Autodesk Inventor part; units mm, degrees
ref_plane "YZ Plane" through (0, 0, 0) normal (1, 0, 0) x (0, 1, 0)
ref_plane "XZ Plane" through (0, 0, 0) normal (0, 1, 0) x (-1, 0, 0)
ref_plane "XY Plane" through (0, 0, 0) normal (0, 0, 1) x (1, 0, 0)
sketch "スケッチ1" plane through (0, 0, 0) normal (1, 0, 0) x (0, 1, 0)
  point P0 (0, 0)
sketch "スケッチ2" plane through (0, 0, 0) normal (0, 0, 1) x (1, 0, 0)
  line L0 (-11.1, 11.1) -> (11.1, 11.1)
  line L1 (11.1, 11.1) -> (11.1, -11.1)
  line L2 (11.1, -11.1) -> (-11.1, -11.1)
  line L3 (-11.1, -11.1) -> (-11.1, 11.1)
  line L4 (-11.1, 11.1) -> (11.1, -11.1) construction
  line L5 (11.1, 11.1) -> (-11.1, -11.1) construction
  line L6 (-13.5, -13.5) -> (13.5, -13.5)
  line L7 (13.5, -13.5) -> (13.5, 13.5)
  line L8 (13.5, 13.5) -> (-13.5, 13.5)
  line L9 (-13.5, 13.5) -> (-13.5, -13.5)
  line L10 (-13.5, -13.5) -> (13.5, 13.5) construction
  line L11 (13.5, -13.5) -> (-13.5, 13.5) construction
  point P0 (0, 0)
  dimension "d0" = 22.2
  dimension "d1" = 22.2
  dimension "d2" = 27
  dimension "d3" = 27
extrude "押し出し1" add sketch "スケッチ2" along normal blind 15
sketch "スケッチ3" plane through (-13.5, 13.5, 0) normal (0, 1, 0) x (1, 0, 0)
  circle A0 centre (13.5, -10) radius 1.7
  point P0 (13.5, 0)
  dimension "d6" = 3.4
extrude "押し出し2" cut sketch "スケッチ3" against normal blind 30
sketch "スケッチ4" plane through (0, 0, 0) normal (0, 0, -1) x (-1, 0, 0)
  line L0 (22, 22) -> (-22, 22)
  line L1 (-22, 22) -> (-22, -22)
  line L2 (-22, -22) -> (22, -22)
  line L3 (22, -22) -> (22, 22)
  line L4 (22, 22) -> (-22, -22) construction
  line L5 (-22, 22) -> (22, -22) construction
  point P0 (0, 0)
  dimension "d9" = 44
  dimension "d10" = 44
extrude "押し出し3" add sketch "スケッチ4" along normal blind 3
sketch "スケッチ5" plane through (0, 0, 0) normal (0, 0, 1) x (1, 0, 0)
  circle A0 centre (0, 17.75) radius 2.25
  circle A1 centre (0, -17.75) radius 2.25
  point P0 (0, 0)
  dimension "d13" = 4.5
  dimension "d14" = 4.5
extrude "押し出し4" cut sketch "スケッチ5" against normal blind 3
sketch "スケッチ6" plane through (0, 0, 0) normal (0, 0, 1) x (1, 0, 0)
  line L0 (-22, 22) -> (22, 22)
  line L1 (22, 22) -> (11, 22)
  line L2 (22, 22) -> (22, 11)
  line L3 (22, 11) -> (11, 22)
  line L4 (22, -22) -> (-22, -22)
  line L5 (22, -22) -> (22, -11)
  line L6 (22, 22) -> (22, -22)
  line L7 (22, -22) -> (11, -22)
  line L8 (11, -22) -> (22, -11)
  line L9 (-22, -22) -> (-22, 22)
  line L10 (-22, 22) -> (-11, 22)
  line L11 (-22, 22) -> (-22, 11)
  line L12 (-22, 11) -> (-11, 22)
  line L13 (-22, -22) -> (-22, -11)
  line L14 (-22, -22) -> (-11, -22)
  line L15 (-22, -11) -> (-11, -22)
  point P0 (0, 0)
  dimension "d17" = 11
  dimension "d18" = 11
  dimension "d19" = 11
  dimension "d20" = 11
  dimension "d21" = 11
  dimension "d22" = 11
  dimension "d23" = 11
extrude "押し出し5" cut sketch "スケッチ6" against normal blind 3 contours L0 L12 L9 | L0 L2 L3 | L15 L4 L9 | L5 L4 L8
fillet "フィレット1" radius 3 4 edges at (13.5, -13.5, 7.5) (13.5, 13.5, 7.5) (-13.5, -13.5, 7.5) (-13.5, 13.5, 7.5)
fillet "フィレット2" radius 1 4 edges at (-11.1, 11.1, 7.5) (-11.1, -11.1, 7.5) (11.1, 11.1, 7.5) (11.1, -11.1, 7.5)
properties part number "rod_fixture_vp16"
Design review of the part built by this model. Coordinates are the model's own, in mm. A direction names the side the tool comes from. Round coordinates to 2 decimals unless told otherwise and drop trailing zeros. Write each loop counter-clockwise with the first axis right and the second up, starting at its lowest first coordinate (ties: lowest second). Pieces come first, ordered by that corner, then holes. Notation, with made-up numbers: (81, 33.5) -> (116, 33.5) arc R22 ccw to (116, 68.5) -> close; hole circle Ø1 at (82, -8). An arc over 180 degrees is marked (long way). One line per question, with ' | ' between items.
(1) Take a section at A-A, the plane x = 0. State the section outline as (y, z) points, and give its area (3 significant figures).
Result sheet:
outline: (-22, -3) -> (-20, -3) -> (-20, 0) -> (-22, 0) -> close; (-15.5, -3) -> (15.5, -3) -> (15.5, 0) -> (13.5, 0) -> (13.5, 8.3) -> (11.1, 8.3) -> (11.1, 0) -> (-11.1, 0) -> (-11.1, 8.3) -> (-13.5, 8.3) -> (-13.5, 0) -> (-15.5, 0) -> close; (-13.5, 11.7) -> (-11.1, 11.7) -> (-11.1, 15) -> (-13.5, 15) -> close; (11.1, 11.7) -> (13.5, 11.7) -> (13.5, 15) -> (11.1, 15) -> close; (20, -3) -> (22, -3) -> (22, 0) -> (20, 0) -> close | area: 161 mm2
(2) Insertion check: P1, Ø4, axis at y = -8.5, z = 11.5, coming from the +X side; P2, Ø5, axis at x = 9, z = 4, coming from the +Y side; P3, Ø4.5, axis at y = -3, z = 8, coming from the -X side. Each pin has a flat end and moves straight along its axis. Give the tip position at first contact, or say it passes through.
Result sheet:
P1: x = 13.5 | P2: y = 13.5 | P3: x = -13.5
(3) Take a section at D-D, the plane z = 10. State the section outline as (x, y) points, and give its area (3 significant figures).
Result sheet:
outline: (-13.5, -10.5) arc R3 ccw to (-10.5, -13.5) -> (-1.7, -13.5) -> (-1.7, -11.1) -> (-10.1, -11.1) arc R1 cw to (-11.1, -10.1) -> (-11.1, 10.1) arc R1 cw to (-10.1, 11.1) -> (-1.7, 11.1) -> (-1.7, 13.5) -> (-10.5, 13.5) arc R3 ccw to (-13.5, 10.5) -> close; (1.7, -13.5) -> (10.5, -13.5) arc R3 ccw to (13.5, -10.5) -> (13.5, 10.5) arc R3 ccw to (10.5, 13.5) -> (1.7, 13.5) -> (1.7, 11.1) -> (10.1, 11.1) arc R1 cw to (11.1, 10.1) -> (11.1, -10.1) arc R1 cw to (10.1, -11.1) -> (1.7, -11.1) -> close | area: 213 mm2
(4) Wall thickness on line 1 (Y direction, x = 0, z = -1.5); line 2 (X direction, y = 2, z = 6.75); line 3 (Z direction, x = 0, y = -11.65): over which ranges is each line inside the solid? List them lowest first. Write a range as [from, to].
Result sheet:
line 1: [-22, -20], [-15.5, 15.5], [20, 22] | line 2: [-13.5, -11.1], [11.1, 13.5] | line 3: [-3, 8.3], [11.7, 15]
(5) Take a section at C-C, the plane z = 1.5. State the section outline as (x, y) points, and give its area (3 significant figures).
Result sheet:
outline: (-13.5, -10.5) arc R3 ccw to (-10.5, -13.5) -> (10.5, -13.5) arc R3 ccw to (13.5, -10.5) -> (13.5, 10.5) arc R3 ccw to (10.5, 13.5) -> (-10.5, 13.5) arc R3 ccw to (-13.5, 10.5) -> close; hole (-11.1, -10.1) arc R1 ccw to (-10.1, -11.1) -> (10.1, -11.1) arc R1 ccw to (11.1, -10.1) -> (11.1, 10.1) arc R1 ccw to (10.1, 11.1) -> (-10.1, 11.1) arc R1 ccw to (-11.1, 10.1) -> close | area: 229 mm2
(6) Machinability: for faces 1 (the flat face through (-13.5, 0, 7)), 2 (the flat face through (13.5, 0, 7)), 3 (the flat face through (0, -13.5, 7)), 4 (the cylindrical face through (-12.64, -12.6, 7.6)), 5 (the flat face through (0, 0, 0)), which of the approach directions +Z, -Z, +X, -X, +Y, -Y give a long, thin tool a straight path to every point of the face, cutting with its end or side? Answer none if there is none.
Result sheet:
face 1: +Z, -X, +Y, -Y | face 2: +Z, +X, +Y, -Y | face 3: +Z, +X, -X, -Y | face 4: +Z, -X, -Y | face 5: +Z
(7) Draft analysis for pull direction Y (two halves, no side actions). For faces 6 (the flat face through (0, -22, -1)), 7 (the cylindrical face through (-10.799, 10.815, 7.605)), 8 (the cylindrical face through (-12.6, 12.64, 7.6)), state which applies: released by +Y, released by -Y, zero draft, split by the parting line, or undercut.
Result sheet:
face 6: released by -Y | face 7: undercut | face 8: released by +Y
(8) Take a section at B-B, the plane y = -17.75. State the section outline as (x, z) points, and give its area (3 significant figures).
Result sheet:
outline: (-15.25, -3) -> (-2.25, -3) -> (-2.25, 0) -> (-15.25, 0) -> close; (2.25, -3) -> (15.25, -3) -> (15.25, 0) -> (2.25, 0) -> close | area: 78.0 mm2
